Read the model definition and answer for the solid it produces. Units are mm, in the model's axes. A direction names the side the tool comes from. Give positions to 0.01 mm unless a question says otherwise; leave off trailing zeros. Loops run counter-clockwise (first coordinate to the right, second up) from the corner with the lowest first, then second, coordinate; pieces in that order, holes last.
(1) Find section D-D, the plane z = 5. Write down the section's boundary in (x, y), then the cut area to 3 significant figures.
(2) Which of the six approach directions +Z, -Z, +X, -X, +Y, -Y give full straight-line access (tool end or side, diameter ignored) to faces 1 (the face through (-0.493, -3.905, 0.867)), 2 (the face through (1.972, -2.787, 7.706)), 3 (the face through (1.54, -5.73, 8.37))?
(3) Each of these flat-tipped pins is pushed along its axis until it touches: P1, Ø1.5, axis at x = 0, y = 5, coming from the +Z side; P2, Ø0.6, axis at y = 3.5, z = 1, coming from the -X side; P3, Ø1, axis at y = 0.5, z = -9, coming from the +X side. Where does it stop, or does it pass through?
(4) Find section B-B, the plane x = 1.75. Write down the section's boundary in (y, z), then the cut area to 3 significant figures.
(5) Find section A-A, the plane y = 0. Write down the section's boundary in (x, z).
(6) Straight lines are drawn through the part: probe 1 along Y at (x, z) = (-0.65, 0); probe 2 along Y at (x, z) = (0.15, 6); probe 3 along X at (y, z) = (2, -11). For each, find the intervals that lie inside material, in ascending order.
(7) Determine the mould class of faces 4 (the face through (4, 5, 0)), 5 (the face through (0, 0, 9)), 6 (the face through (1.54, -5.77, -8.13)) for opening direction Z: pulls with the +Z half, pulls with the -Z half, needs draft (parallel to the pull), parting line crosses it, or undercut.
(8) Find section C-C, the plane z = -3. Write down the section's boundary in (x, y).
```python
from build123d import *

# Parameters (mm, degrees)
BOSS_EXTRUDE1_DEPTH = 4
SKETCH2_R           = 4
BOSS_EXTRUDE2_DEPTH = 1


with BuildPart() as part:
    # Sketch1 → Boss-Extrude1 (new body)
    with BuildSketch(Plane(origin=(0, 0, 0), x_dir=(0, 0, -1), z_dir=(1, 0, 0))):
        with BuildLine():
            Line((0, 7), (-16.2, 4.5))
            ThreePointArc((-16.2, 4.5), (-18.456321812, 0.070210727), (-16.5, -4.5))
            Line((-16.5, -4.5), (0, -7))
            Line((0, -7), (16.5, -4.5))
            ThreePointArc((16.5, -4.5), (18.456321812, 0.070210727), (16.2, 4.5))
            Line((16.2, 4.5), (0, 7))
        make_face()
        with BuildLine():
            Line((0, 3.7), (-15.2, 1.9))
            ThreePointArc((-15.2, 1.9), (-16.123290742, 0), (-15.2, -1.9))
            Line((-15.2, -1.9), (0, -3.7))
            Line((0, -3.7), (15.2, -1.9))
            ThreePointArc((15.2, -1.9), (16.123290742, 0), (15.2, 1.9))
            Line((15.2, 1.9), (0, 3.7))
        make_face(mode=Mode.SUBTRACT)
    extrude(amount=BOSS_EXTRUDE1_DEPTH)

    # Sketch2 → Boss-Extrude2 (add)
    with BuildSketch(Plane(origin=(0, 0, 0), x_dir=(0, 0, -1), z_dir=(1, 0, 0))):
        with BuildLine():
            Line((0, 7), (-16.2, 4.5))
            ThreePointArc((-16.2, 4.5), (-18.456321812, 0.070210727), (-16.5, -4.5))
            Line((-16.5, -4.5), (0, -7))
            Line((0, -7), (16.5, -4.5))
            ThreePointArc((16.5, -4.5), (18.456321812, 0.070210727), (16.2, 4.5))
            Line((16.2, 4.5), (0, 7))
        make_face()
        Circle(SKETCH2_R, mode=Mode.SUBTRACT)
    extrude(amount=-BOSS_EXTRUDE2_DEPTH)


solid = part.part
```
Entries:
1. outline: (-1, -6.24) - (4, -6.24) - (4, -3.11) - (0, -3.11) - (0, 3.11) - (4, 3.11) - (4, 6.23) - (-1, 6.23) - close
1. area: 37.5 mm2
2. face 1: -X
2. face 2: +X
2. face 3: +Z, +X, -X, -Y
3. P1: stops at z = 16.5
3. P2: stops at x = 0
3. P3: stops at x = 0
4. outline: (-7, 0) - (-4.5, -16.5) arc R5.86 ccw to (4.5, -16.2) - (7, 0) - (4.5, 16.2) arc R5.86 ccw to (-4.5, 16.5) - close; hole (-3.7, 0) - (-1.9, -15.2) arc R2.42 ccw to (1.9, -15.2) - (3.7, 0) - (1.9, 15.2) arc R2.42 ccw to (-1.9, 15.2) - close
4. area: 227 mm2
5. outline: (-1, -18.46) - (4, -18.46) - (4, -16.12) - (0, -16.12) - (0, -4) - (-1, -4) - close; (-1, 4) - (0, 4) - (0, 16.12) - (4, 16.12) - (4, 18.46) - (-1, 18.46) - close
6. probe 1: y = -7 to -4, 4 to 7
6. probe 2: y = -6.09 to -2.99, 2.99 to 6.07
6. probe 3: x = -1 to 0
7. face 4: needs draft
7. face 5: undercut
7. face 6: pulls with the -Z half
8. outline: (-1, -6.55) - (4, -6.55) - (4, -3.34) - (0, -3.34) - (0, -2.65) - (-1, -2.65) - close; (-1, 2.65) - (0, 2.65) - (0, 3.34) - (4, 3.34) - (4, 6.54) - (-1, 6.54) - close
